Geometry: final body of the model. Coordinates: model frame, mm. A direction names the side the tool comes from. Coordinates: 2 decimals unless noted, no trailing zeros. Order: outer loops, then holes, each group sorted by start corner. A loop starts at its lowest first (then second) coordinate and runs counter-clockwise, first axis right, second up. Notation, with made-up numbers: M -26,74.5 L 28,74.5 A20 ccw 28,84.5 Z; hole C 84.25,26.5 d4. An arc over 180 degrees is marked long. Use CSV: the item, a comma, the result in double quotes. Start each with the question number.
1. Material intervals for line 1 (Y direction, x = 2.85, z = -5); line 2 (Z direction, x = 2.4, y = 10); line 3 (Z direction, x = -74.5, y = 1), sorted ascending.
2. Section query B-B on y = 16.25. Return the cut outline in (x, z) (3 decimals), and give its area (3 significant figures).
3. Section query A-A on z = 4.25. Return the cut outline in (x, y).
4. Pull-direction query (X, two-part tool) for faces 4 (the flat face through (4, 10, 13)), 5 (the flat face through (-138.262, 8, 5)), 6 (the flat face through (-135.27, 7.46, 2.52)); classes: pulls with the +X half, pulls with the -X half, needs draft (parallel to the pull), parting line crosses it, or undercut.
5. Section query C-C on x = -113.5. Return the cut outline in (y, z).
6. First-contact query: P1, Ø6, axis at y = 10, z = -6.5, coming from the +X side; P2, Ø1, axis at x = -78.5, z = 4.5, coming from the +Y side; P3, Ø3, axis at x = -122.5, y = 11, coming from the +Z side. Flat tips, straight axial feed; report the tip coordinate or a pass-through.
7. Set-up query: faces 1 (the flat face through (5, 10, 0)), 2 (the flat face through (-70, 10, 5)), 3 (the flat face through (-67, 5, 10)). Return all of +Z, -Z, +X, -X, +Y, -Y with unobstructed straight access to the full face (end or side cutting, diameter ignored); none if empty.
Autodesk Fusion 360 part; units mm, degrees
sketch "Sketch1" plane through (0, 0, 0) normal (0, 1, 0) x (1, 0, 0)
  line L0 (0, 0) -> (-25, 0)
  line L1 (-25, 0) -> (-25, -5)
  line L2 (-25, -5) -> (5, -5)
  line L3 (0, 0) -> (0, 10)
  line L4 (0, 10) -> (5, 10)
  line L5 (5, 10) -> (5, -5)
  line L6 (-25, 0) -> (-245, 0)
  line L7 (-245, 0) -> (-245, -5)
  line L8 (-245, -5) -> (-25, -5)
  line L9 (-25, 0) -> (-140, 0)
  line L10 (-140, 0) -> (-140, 27.0089)
  line L11 (-270, 10) -> (-275, 10)
  line L12 (-270, 0) -> (-270, 10)
  line L13 (-275, 10) -> (-275, -5)
  line L14 (-270, 0) -> (-245, 0)
  line L15 (-245, -5) -> (-275, -5)
  line L16 (-245, 0) -> (-245, -5)
  point P0 (-270, 0)
  dimension "d1" = 25
  dimension "d2" = 5
  dimension "d3" = 30
  dimension "d4" = 10
  dimension "d5" = 5
  dimension "d6" = 220
  dimension "d7" = 5
  dimension "d8" = 115
extrude "Extrude1" add sketch "Sketch1" along normal blind 10
extrude "Extrude2" add sketch "Sketch1" along normal blind 20 contours L0 L1 L2 L3 L4 L5 | L7 L11 L12 L13 L14 L15 L16
sketch "Sketch2" plane through (5, 0, 0) normal (1, 0, 0) x (0, 0, -1)
  line L0 (-5, 0) -> (10, 0)
  line L1 (10, 0) -> (10, 20)
  line L2 (10, 20) -> (-5, 20)
  line L3 (-5, 20) -> (-5, 0)
sketch "Sketch3" plane through (0, 0, 0) normal (-1, 0, 0) x (0, 0, 1)
  line L0 (-10, 0) -> (0, 0)
  line L1 (0, 0) -> (0, 20)
  line L2 (0, 20) -> (-10, 20)
  line L3 (-10, 20) -> (-10, 0)
  line L4 (-10, 0) -> (-5, 0)
  line L5 (-5, 0) -> (-5, 10)
  circle A0 centre (-5, 10) radius 2.25
  dimension "d13" = 5
  dimension "d14" = 10
  dimension "d15" = 4.5
extrude "Extrude3" cut sketch "Sketch3" along normal mid plane 662 contours A0
chamfer "Chamfer1" distance 5 angle 45 4 edges at (2.5, 20, -10) (2.5, 0, -10) (-272.5, 20, -10) (-272.5, 0, -10)
sketch "Sketch5" plane through (0, 10, 0) normal (0, 1, 0) x (-1, 0, 0)
  line L0 (25, 5) -> (25, 0)
  line L1 (25, 0) -> (245, 0)
  line L2 (245, 0) -> (245, 5)
  line L3 (245, 5) -> (25, 5)
  line L4 (245, 0) -> (135, 0)
  dimension "d30" = 110
sketch "Sketch6" plane through (0, 0, 5) normal (0, 0, 1) x (1, 0, 0)
  line L0 (-25, 10) -> (-245, 10)
  line L1 (-245, 10) -> (-245, 20)
  line L2 (-245, 20) -> (-275, 20)
  line L3 (-275, 20) -> (-275, 0)
  line L4 (-275, 0) -> (5, 0)
  line L5 (5, 0) -> (5, 20)
  line L6 (5, 20) -> (-25, 20)
  line L7 (-25, 20) -> (-25, 10)
extrude "Extrude5" add 1 faces at (-265, 10, 5) along direction (0, 0, 1) blind 5
sketch "Sketch7" plane through (0, 10, 0) normal (0, 1, 0) x (-1, 0, 0)
  line L0 (25, 10) -> (25, 0)
  line L1 (25, 0) -> (245, 0)
  line L2 (245, 0) -> (245, 10)
  line L3 (245, 10) -> (25, 10)
  line L4 (245, 0) -> (135, 0)
  line L5 (138.2622, 1.9923) -> (132.3533, 3.0342)
  line L6 (138.2622, 7.9923) -> (132.3533, 6.9504)
  line L7 (132.3533, 3.0342) -> (132.3533, 0)
  line L8 (138.2622, 7.9923) -> (138.2622, 1.9923)
  line L9 (132.3533, 6.9504) -> (132.3533, 10)
  line L10 (138.2622, 1.9923) -> (141.0619, 1.9923) construction
  line L11 (138.2622, 7.9923) -> (141.0619, 7.9923) construction
  line L12 (25, 0) -> (245, 0)
  line L13 (128.521, 0) -> (128.521, 5)
  line L14 (270, -5) -> (275, -5)
  line L15 (275, -5) -> (275, 10)
  line L16 (275, 10) -> (245, 10)
  line L17 (245, 10) -> (245, 0)
  line L18 (245, 0) -> (270, 0)
  line L19 (270, 0) -> (270, -5)
  point P0 (132.1074, 10.0354)
  point P1 (138.2622, 4.9923)
  dimension "d33" = 110
  dimension "d34" = 6
  dimension "d35" = 170
  dimension "d36" = 6
  dimension "d37" = 170
  dimension "d38" = 6
  dimension "d41" = 5
extrude "Extrude6" cut sketch "Sketch7" against normal blind 5 contours L1 L2 L3 L4 L5 L6 L7 L8 L9 L12 L17
sketch "Sketch8" plane through (0, 5, 0) normal (0, 1, 0) x (-1, 0, 0)
  line L0 (138.2622, 7.9923) -> (138.2622, 1.9923)
  line L1 (138.2622, 1.9923) -> (132.3533, 3.0342)
  line L2 (132.3533, 3.0342) -> (132.3533, 0)
  line L3 (132.3533, 0) -> (245, 0)
  line L4 (245, 0) -> (245, 10)
  line L5 (245, 10) -> (132.3533, 10)
  line L6 (132.3533, 10) -> (132.3533, 6.9504)
  line L7 (132.3533, 6.9504) -> (138.2622, 7.9923)
  line L8 (245, 5) -> (25, 5)
  line L9 (270, -5) -> (275, -5)
  line L10 (275, -5) -> (275, 10)
  line L11 (275, 10) -> (245, 10)
  line L12 (245, 10) -> (245, 0)
  line L13 (245, 0) -> (270, 0)
  line L14 (270, 0) -> (270, -5)
  line L15 (275, -10) -> (275, -5)
  line L16 (275, -5) -> (270, -5)
  line L17 (270, -5) -> (270, -10)
  line L18 (270, -10) -> (275, -10)
  line L19 (138.2622, 1.9923) -> (138.2622, 0)
  line L20 (138.2622, 0) -> (132.3533, 0)
  line L21 (132.3533, 3.0342) -> (132.3533, 0)
  line L22 (138.2622, 7.9923) -> (138.2622, 10)
sketch "Sketch9" plane through (0, 20, 0) normal (0, 1, 0) x (-1, 0, 0)
  line L0 (270, -5) -> (275, -5)
  line L1 (275, -5) -> (275, 10)
  line L2 (275, 10) -> (245, 10)
  line L3 (245, 10) -> (245, 0)
  line L4 (245, 0) -> (270, 0)
  line L5 (270, 0) -> (270, -5)
  line L6 (275, -10) -> (275, -5)
  line L7 (275, -5) -> (270, -5)
  line L8 (270, -5) -> (270, -10)
  line L9 (270, -10) -> (275, -10)
  line L10 (138.2622, 7.9923) -> (138.2622, 1.9923)
  line L11 (138.2622, 1.9923) -> (132.3533, 3.0342)
  line L12 (132.3533, 3.0342) -> (132.3533, 0)
  line L13 (132.3533, 0) -> (245, 0)
  line L14 (245, 0) -> (245, 10)
  line L15 (245, 10) -> (132.3533, 10)
  line L16 (132.3533, 10) -> (132.3533, 6.9504)
  line L17 (132.3533, 6.9504) -> (138.2622, 7.9923)
  line L18 (138.2622, 1.9923) -> (138.2622, -2.244)
  line L19 (138.2622, -2.244) -> (138.2622, 11)
extrude "Extrude7" cut sketch "Sketch9" against normal blind 40 contours L0 L1 L2 L3 L4 L5 L7 L14 | L0 L6 L7 L8 L9 | L3 L10 L13 L14 L15 L18 L19
sketch "Sketch10" plane through (0, 10, 0) normal (0, 1, 0) x (-1, 0, 0)
  line L0 (132.3533, 0) -> (132.3533, 3.0342)
  line L1 (132.3533, 3.0342) -> (138.2622, 1.9923)
  line L2 (138.2622, 1.9923) -> (138.2622, 7.9923)
  line L3 (138.2622, 7.9923) -> (132.3533, 6.9504)
  line L4 (132.3533, 6.9504) -> (132.3533, 10)
  line L5 (132.3533, 10) -> (25, 10)
  line L6 (25, 10) -> (25, 0)
  line L7 (25, 0) -> (132.3533, 0)
sketch "Sketch11" plane through (0, 0, 0) normal (0, -1, 0) x (1, 0, 0)
  line L0 (-138.2622, 10) -> (-138.2622, 0)
  line L1 (-138.2622, 0) -> (0, 0)
  line L2 (0, 0) -> (0, -5)
  line L3 (0, -5) -> (5, -5)
  line L4 (5, -5) -> (5, 10)
  line L5 (5, 10) -> (-138.2622, 10)
  line L6 (-132.3533, 0) -> (-132.3533, 3.0342)
  line L7 (-132.3533, 3.0342) -> (-138.2622, 1.9923)
  line L8 (-138.2622, 1.9923) -> (-138.2622, 7.9923)
  line L9 (-138.2622, 7.9923) -> (-132.3533, 6.9504)
  line L10 (-132.3533, 6.9504) -> (-132.3533, 10)
  line L11 (-132.3533, 10) -> (-25, 10)
  line L12 (-25, 10) -> (-25, 0)
  line L13 (-25, 0) -> (-132.3533, 0)
  line L14 (-138.2622, 7.9923) -> (-138.2622, 10)
  line L15 (-132.3533, 10) -> (-132.3533, 0)
  line L16 (-138.2622, 0) -> (-138.2622, 1.9923)
  line L17 (-138.2622, 0) -> (-132.3533, 0)
extrude "Extrude8" cut sketch "Sketch11" against normal blind 10 contours L0 L5 L9 L10 L14 L15
extrude "Extrude9" cut sketch "Sketch11" against normal blind 9 contours L0 L1 L6 L7 L15 L16 L17
extrude "Extrude10" cut sketch "Sketch11" against normal blind 5 contours L0 L7 L8 L9 L15
sketch "Sketch12" plane through (0, 20, 0) normal (0, 1, 0) x (-1, 0, 0)
  line L0 (-5, -5) -> (0, -5)
  line L1 (0, -5) -> (0, 0)
  line L2 (0, 0) -> (25, 0)
  line L3 (25, 0) -> (25, 10)
  line L4 (25, 10) -> (-5, 10)
  line L5 (-5, 10) -> (-5, -5)
  line L6 (0, 0) -> (25, 0)
  line L7 (25, 0) -> (25, 10)
  line L8 (25, 10) -> (0, 10)
  line L9 (0, 10) -> (0, 0)
extrude "Extrude11" cut sketch "Sketch12" against normal blind 10 contours L2 L3 L4 L6 L7 L8 L9
sketch "Sketch13" plane through (0, 0, 10) normal (0, 0, 1) x (1, 0, 0)
  line L0 (0, 10) -> (-132.3533, 10)
  line L1 (-132.3533, 10) -> (-132.3533, 0)
  line L2 (-132.3533, 0) -> (5, 0)
  line L3 (5, 0) -> (5, 20)
  line L4 (5, 20) -> (0, 20)
  line L5 (0, 20) -> (0, 10)
  line L6 (0, 0) -> (8.175, 0)
  line L7 (0, 20) -> (0, 0)
  line L8 (0, 20) -> (8.175, 20)
  line L9 (8.175, 20) -> (8.175, 0)
  dimension "d56" = 8.175
extrude "Extrude12" add sketch "Sketch13" along normal blind 3 contours L2 L3 L4 L5 L6 L7 L8 | L3 L6 L8 L9
extrude "Extrude13" cut 1 faces at (8.175, 13.3333, 11) along direction (-1, 0, 0) blind 0.5
equation "d56 = 5 mm + ( 25.4 / 8 ) * 1 mm"
Results list:
1,line 1,"y = 0 to 7.75, 12.25 to 20"
1,line 2,"z = -10 to -7.25, -2.75 to 13"
1,line 3,"z = 0 to 10"
2,outline,"M 0,-8.75 L 5,-8.75 L 5,10 L 7.675,10 L 7.675,13 L 0,13 Z"
2,area,"117 mm²"
3,outline,"M -138.26,5 L -132.35,5 L -132.35,0 L 5,0 L 5,20 L 0,20 L 0,10 L -138.26,10 Z"
4,face 4,"needs draft"
4,face 5,"pulls with the -X half"
4,face 6,"undercut"
5,outline,"M 0,0 L 10,0 L 10,10 L 0,10 Z"
6,P1,"stops at x = 5"
6,P2,"stops at y = 10"
6,P3,"stops at z = 10"
7,face 1,"-Z, +X, +Y, -Y"
7,face 2,"+Z, -Z, -X, +Y"
7,face 3,"+Z, -X, +Y, -Y"
